```python
from build123d import *

# Parameters (mm, degrees)
SKETCH_1_R          = 45
EXTRUDE_1_DEPTH     = 10
SKETCH_2_R          = 10
SKETCH_2_R_2        = 3.25
SKETCH_2_R_3        = 2.5
CUT_EXTRUDE_1_DEPTH = 11


with BuildPart() as part:
    # 草图1 → 凸台-拉伸1 (new body)
    with BuildSketch(Plane.XY):
        Circle(SKETCH_1_R)
    extrude(amount=EXTRUDE_1_DEPTH)

    # 草图2 → 切除-拉伸1 (cut)
    with BuildSketch(Plane(origin=(0, 0, 0), x_dir=(-1, 0, 0), z_dir=(0, 0, -1))):
        Circle(SKETCH_2_R)
        with Locations((-22, 0)):
            Circle(SKETCH_2_R_2)
        with Locations((-11, 19.052558883)):
            Circle(SKETCH_2_R_2)
        with Locations((11, 19.052558883)):
            Circle(SKETCH_2_R_2)
        with Locations((22, 0)):
            Circle(SKETCH_2_R_2)
        with Locations((11, -19.052558883)):
            Circle(SKETCH_2_R_2)
        with Locations((-11, -19.052558883)):
            Circle(SKETCH_2_R_2)
        with Locations((-22.627416998, 22.627416998)):
            Circle(SKETCH_2_R_3)
        with Locations((22.627416998, 22.627416998)):
            Circle(SKETCH_2_R_3)
        with Locations((22.627416998, -22.627416998)):
            Circle(SKETCH_2_R_3)
        with Locations((-22.627416998, -22.627416998)):
            Circle(SKETCH_2_R_3)
    extrude(amount=-CUT_EXTRUDE_1_DEPTH, mode=Mode.SUBTRACT)


solid = part.part
```
Check sheet for the modelled part. Datum: model origin and axes. Units: mm. Give positions to 0.01 mm unless a question says otherwise; leave off trailing zeros. Order: outer loops, then holes, each group sorted by start corner. A loop starts at its lowest first (then second) coordinate and runs counter-clockwise, first axis right, second up. Notation, with made-up numbers: M 40,29.25 L 78,29.25 A24 ccw 78,55.25 Z; hole C 84.5,56.5 d2. An arc over 180 degrees is marked long. Answer in a Markdown table with one row per item.
1) Cross-section at B-B, the plane y = 0. Enter the section's corners in (x, z).
Filled sheet:
| item | result |
|---|---|
| outline | M -45,0 L -25.25,0 L -25.25,10 L -45,10 Z; M -18.75,0 L -10,0 L -10,10 L -18.75,10 Z; M 10,0 L 18.75,0 L 18.75,10 L 10,10 Z; M 25.25,0 L 45,0 L 45,10 L 25.25,10 Z |
2) Cross-section at A-A, the plane x = 0. Enter the section's corners in (y, z), plus the area to 3 significant figures.
Filled sheet:
| item | result |
|---|---|
| outline | M -45,0 L -10,0 L -10,10 L -45,10 Z; M 10,0 L 45,0 L 45,10 L 10,10 Z |
| area | 700 mm2 |
3) Thickness scan on L1, parallel to Y at x = -11, z = 7.25; L2, parallel to Y at x = -22, z = 4.25; L3, parallel to X at y = -22.5, z = 3.25. Record the ranges inside material, lowest first. Write a range as [from, to].
Filled sheet:
| item | result |
|---|---|
| L1 | y = [-43.63, -22.3], [-15.8, 15.8], [22.3, 43.63] |
| L2 | y = [-39.26, -25.05], [-20.21, -3.25], [3.25, 20.21], [25.05, 39.26] |
| L3 | x = [-38.97, -25.12], [-20.13, 20.13], [25.12, 38.97] |
4) Release check for a two-part mould opening along X. For faces 1 (the cylindrical face through (20.765, -39.923, 4.93)), 2 (the cylindrical face through (11.7, 15.88, 4.93)), 3 (the cylindrical face through (-22.09, -25.07, 4.93)), 4 (the flat face through (-1, 11, 0)) record: +X half, -X half, draft (parallel to the pull), parting line (faces both ways), or undercut.
Filled sheet:
| item | result |
|---|---|
| face 1 | parting line |
| face 2 | undercut |
| face 3 | undercut |
| face 4 | draft |
5) Cross-section at C-C, the plane x = 22. Enter the section's corners in (y, z).
Filled sheet:
| item | result |
|---|---|
| outline | M -39.26,0 L -25.05,0 L -25.05,10 L -39.26,10 Z; M -20.21,0 L -3.25,0 L -3.25,10 L -20.21,10 Z; M 3.25,0 L 20.21,0 L 20.21,10 L 3.25,10 Z; M 25.05,0 L 39.26,0 L 39.26,10 L 25.05,10 Z |
6) Cross-section at D-D, the plane z = 8.75. Count the separate pieces of the cut face and the enclosed holes in it, plus the area to 3 significant figures.
Filled sheet:
| item | result |
|---|---|
| separate pieces | 1 |
| enclosed holes | 11 |
| area | 5,770 mm2 |
7) Gauge pin test, flat ends, axial feed: P1, Ø8, axis at x = 23.5, y = 11, coming from the -Z side; P2, Ø5, axis at y = -28.5, z = 2, coming from the -X side; P3, Ø5, axis at x = 8.5, z = 6.5, coming from the -Y side. Record the tip position at first contact, or that the pin passes through.
Filled sheet:
| item | result |
|---|---|
| P1 | stops at z = 0 |
| P2 | stops at x = -36.73 |
| P3 | stops at y = -44.6 |
